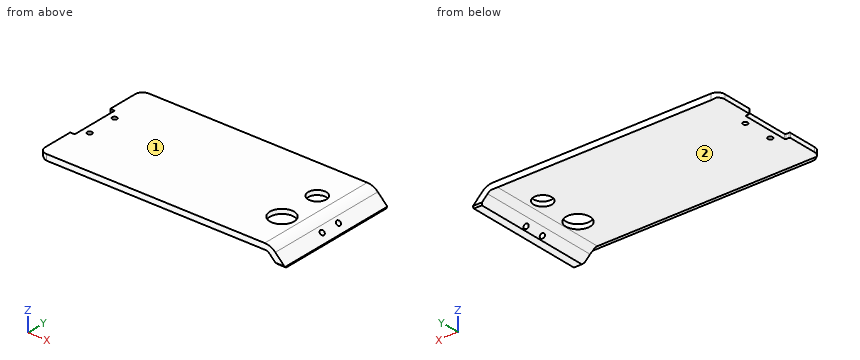
from build123d import *

# Parameters (mm, degrees)
SKETCH_1_W            = 88.2
SKETCH_1_H            = 177
EXTRUDE_1_DEPTH       = 52.9
SHELL_1_T             = -3
CUT_EXTRUDE_5_REACH   = 206.711
SKETCH_16_R           = 6.05
SKETCH_16_R_2         = 8.05
CHAMFER_7_SIZE        = 10
CHAMFER_8_SIZE        = 1
SKETCH_21_W           = 10.5
SKETCH_21_H           = 82.2
EXTRUDE_7_DEPTH       = 6
SKETCH_22_OUTSIDE_W   = 219.942
SKETCH_22_OUTSIDE_H   = 131.142
SKETCH_22_OUTSIDE_W_2 = 164.4
SKETCH_22_OUTSIDE_H_2 = 82
CUT_EXTRUDE_8_DEPTH   = 10
SKETCH_23_W           = 177
SKETCH_23_H           = 42.9
CUT_EXTRUDE_9_DEPTH   = 205.711137948
FILLET_3_R            = 10
FILLET_4_R            = 5.1
SKETCH_24_R           = 1.6
CUT_EXTRUDE_10_DEPTH  = 146.652789194
CHAMFER_10_SIZE       = 1
CHAMFER_10_SIZE_2     = 0.707106781
CUT_EXTRUDE_11_REACH  = 198.013
SKETCH_25_R           = 1.6
FILLET_5_R            = 8
CUT_EXTRUDE_12_REACH  = 198.013
SKETCH_26_W           = 3
SKETCH_26_H           = 32
FILLET_6_R            = 0.5


with BuildPart() as part:
    # 草图1 → 凸台-拉伸1 (new body)
    with BuildSketch(Plane(origin=(0, 0, 0), x_dir=(0, 1, 0), z_dir=(0, 0, 1))):
        with Locations((44.1, -88.5)):
            Rectangle(SKETCH_1_W, SKETCH_1_H)
    extrude(amount=EXTRUDE_1_DEPTH)

    # 抽壳1
    shell_1_openings = [part.faces().sort_by_distance(p)[0] for p in [
        (88.5, 44.1, 0),
    ]]
    offset(amount=SHELL_1_T, openings=shell_1_openings, kind=Kind.INTERSECTION)

    # 草图16 → 切除-拉伸5 (cut, up to next)
    with BuildSketch(Plane.XY.offset(52.9), mode=Mode.PRIVATE) as cut_extrude_5_sk1:
        with Locations((152, 58.2)):
            Circle(SKETCH_16_R)
    cut_extrude_5_tool1 = extrude(cut_extrude_5_sk1.sketch, amount=-CUT_EXTRUDE_5_REACH, mode=Mode.PRIVATE) & part.part
    # 草图16 → 切除-拉伸5 (cut, up to next)
    with BuildSketch(Plane.XY.offset(52.9), mode=Mode.PRIVATE) as cut_extrude_5_sk2:
        with Locations((152, 30)):
            Circle(SKETCH_16_R_2)
    cut_extrude_5_tool2 = extrude(cut_extrude_5_sk2.sketch, amount=-CUT_EXTRUDE_5_REACH, mode=Mode.PRIVATE) & part.part
    add(cut_extrude_5_tool1.solids().sort_by_distance((152, 58.2, 52.9))[0], mode=Mode.SUBTRACT)
    add(cut_extrude_5_tool2.solids().sort_by_distance((152, 30, 52.9))[0], mode=Mode.SUBTRACT)

    # 倒角7
    chamfer_7_edges = [part.edges().sort_by_distance(p)[0] for p in [
        (174, 44.1, 49.9),
        (177, 44.1, 52.9),
    ]]
    chamfer(chamfer_7_edges, length=CHAMFER_7_SIZE)

    # 倒角8
    chamfer_8_edges = [part.edges().sort_by_distance(p)[0] for p in [
        (83.5, 3, 49.9),
        (83.5, 88.2, 52.9),
        (177, 88.2, 21.45),
        (172, 88.2, 47.9),
        (177, 0, 21.45),
        (172, 0, 47.9),
        (83.5, 85.2, 49.9),
        (83.5, 0, 52.9),
    ]]
    chamfer(chamfer_8_edges, length=CHAMFER_8_SIZE)

    # 草图21 → 凸台-拉伸7 (add)
    with BuildSketch(Plane(origin=(0, 0, 0), x_dir=(-1, 0, 0), z_dir=(0, 0, -1))):
        with Locations((-168.75, 44.1)):
            Rectangle(SKETCH_21_W, SKETCH_21_H)
        with Locations((-8.25, 44.1)):
            Rectangle(SKETCH_21_W, SKETCH_21_H)
    extrude(amount=-EXTRUDE_7_DEPTH)

    # 草图22 outside → 切除-拉伸8 (cut)
    with BuildSketch(Plane.XY.offset(52.9)):
        with Locations((88.5, 44.1)):
            Rectangle(SKETCH_22_OUTSIDE_W, SKETCH_22_OUTSIDE_H)
        with Locations((94.8, 44.1)):
            Rectangle(SKETCH_22_OUTSIDE_W_2, SKETCH_22_OUTSIDE_H_2, mode=Mode.SUBTRACT)
    extrude(amount=-CUT_EXTRUDE_8_DEPTH, mode=Mode.SUBTRACT)

    # 草图23 → 切除-拉伸9 (cut, through all)
    with BuildSketch(Plane.XZ):
        with Locations((88.5, 21.45)):
            Rectangle(SKETCH_23_W, SKETCH_23_H)
    extrude(amount=-CUT_EXTRUDE_9_DEPTH, mode=Mode.SUBTRACT)

    # 圆角3
    fillet_3_edges = [part.edges().sort_by_distance(p)[0] for p in [
        (167, 44.1, 52.9),
    ]]
    fillet(fillet_3_edges, radius=FILLET_3_R)

    # 圆角4
    fillet_4_edges = [part.edges().sort_by_distance(p)[0] for p in [
        (12.6, 3.1, 50.95),
        (12.6, 85.1, 50.95),
    ]]
    fillet(fillet_4_edges, radius=FILLET_4_R)

    # 草图24 → 切除-拉伸10 (cut, through all)
    with BuildSketch(Plane(origin=(109.95, 0, 109.95), x_dir=(0.7071067811865456, 0, -0.7071067811865495), z_dir=(0.7071067811865495, 0, 0.7071067811865456))):
        with Locations((88.323019357, 50.6)):
            Circle(SKETCH_24_R)
        with Locations((88.323019357, 37.6)):
            Circle(SKETCH_24_R)
    extrude(amount=-CUT_EXTRUDE_10_DEPTH, mode=Mode.SUBTRACT)

    # 倒角10
    # the kernel refuses this chamfer: 1, 0.707106781 mm, written as the material it takes off along each edge
    with BuildSketch(Plane(origin=(177, 87.671682988, 42.9), x_dir=(-0.6873969152646486, 0, 0.7262819568766976), z_dir=(0, -1, 0))) as chamfer_10_piece_1:
        Polygon((CHAMFER_10_SIZE * 0.999621916911, CHAMFER_10_SIZE * 0.0274958766106), (CHAMFER_10_SIZE_2 * 0.687396915446, CHAMFER_10_SIZE_2 * 0.726281957068), (0, 0), align=None)
    extrude(amount=87.143365976, mode=Mode.SUBTRACT)
    with BuildSketch(Plane(origin=(179.571682988, 3.1, 42.9), x_dir=(0, -0.027495876610586414, 0.9996219169112968), z_dir=(-1, 0, 0))) as chamfer_10_piece_2:
        Polygon((CHAMFER_10_SIZE * 0.999621916911, CHAMFER_10_SIZE * 0.0274958766106), (-CHAMFER_10_SIZE * 0.0274958766106, CHAMFER_10_SIZE * 0.999621916911), (0, 0), align=None)
    extrude(amount=11.143365976, mode=Mode.SUBTRACT)
    with BuildSketch(Plane(origin=(168.428317012, 85.1, 42.9), x_dir=(0, -0.9996219169112968, -0.027495876610589196), z_dir=(1, 0, 0))) as chamfer_10_piece_3:
        Polygon((CHAMFER_10_SIZE * 0.999621916911, -CHAMFER_10_SIZE * 0.0274958766106), (-CHAMFER_10_SIZE * 0.0274958766106, -CHAMFER_10_SIZE * 0.999621916911), (0, 0), align=None)
    extrude(amount=11.143365976, mode=Mode.SUBTRACT)

    # 草图25 → 切除-拉伸11 (cut, up to next)
    with BuildSketch(Plane.XY.offset(52.9), mode=Mode.PRIVATE) as cut_extrude_11_sk1:
        with Locations((20.6, 54.1)):
            Circle(SKETCH_25_R)
    cut_extrude_11_tool1 = extrude(cut_extrude_11_sk1.sketch, amount=-CUT_EXTRUDE_11_REACH, mode=Mode.PRIVATE) & part.part
    # 草图25 → 切除-拉伸11 (cut, up to next)
    with BuildSketch(Plane.XY.offset(52.9), mode=Mode.PRIVATE) as cut_extrude_11_sk2:
        with Locations((20.6, 34.1)):
            Circle(SKETCH_25_R)
    cut_extrude_11_tool2 = extrude(cut_extrude_11_sk2.sketch, amount=-CUT_EXTRUDE_11_REACH, mode=Mode.PRIVATE) & part.part
    add(cut_extrude_11_tool1.solids().sort_by_distance((20.6, 54.1, 52.9))[0], mode=Mode.SUBTRACT)
    add(cut_extrude_11_tool2.solids().sort_by_distance((20.6, 34.1, 52.9))[0], mode=Mode.SUBTRACT)

    # 圆角5
    fillet_5_edges = [part.edges().sort_by_distance(p)[0] for p in [
        (164, 44.1, 49.9),
    ]]
    fillet(fillet_5_edges, radius=FILLET_5_R)

    # 草图26 → 切除-拉伸12 (cut, up to next)
    with BuildSketch(Plane.XY.offset(52.9), mode=Mode.PRIVATE) as cut_extrude_12_sk1:
        with Locations((14.1, 44.1)):
            Rectangle(SKETCH_26_W, SKETCH_26_H)
    cut_extrude_12_tool1 = extrude(cut_extrude_12_sk1.sketch, amount=-CUT_EXTRUDE_12_REACH, mode=Mode.PRIVATE) & part.part
    add(cut_extrude_12_tool1.solids().sort_by_distance((14.1, 44.1, 52.9))[0], mode=Mode.SUBTRACT)

    # 圆角6
    fillet_6_edges = [part.edges().sort_by_distance(p)[0] for p in [
        (12.6, 28.1, 51.4),
        (12.6, 60.1, 51.4),
        (15.6, 60.1, 51.4),
        (15.6, 28.1, 51.4),
    ]]
    fillet(fillet_6_edges, radius=FILLET_6_R)


solid = part.part
Read the model definition and answer for the solid it produces. Units are mm, in the model's axes. Face numbers are marked on the shaded views. Coordinates: 2 decimals unless noted, no trailing zeros. Order: outer loops, then holes, each group sorted by start corner. A loop starts at its lowest first (then second) coordinate and runs counter-clockwise, first axis right, second up. Notation, with made-up numbers: M 86,-19 L 94,-19 A22 ccw 94,-7 Z; hole C 47,-3.75 d4. An arc over 180 degrees is marked long. Put each result on its own line as item: value. Start each with the question number.
Item 1: Consider probe 1 along Y at (x, z) = (20.6, 50.7); probe 2 along Y at (x, z) = (152, 50.55); probe 3 along Z at (x, y) = (81, 20). Determine where each line is inside the solid, lowest interval first. Write a range as [from, to].
Item 2: Given pin 1 Ø2.5 at (x, y) = (20.6, 34.1) entering from +Z; pin 2 Ø1 at (x, z) = (14.5, 51) entering from -Y; pin 3 Ø2.5 at (y, z) = (46.5, 52) entering from -X; pin 4 Ø1.6 at (x, z) = (14, 51) entering from +Y, each flat-ended and moving along its own axis, determine where each tip first touches the part or whether it passes through.
Item 3: Section C-C, the plane y = 54.1 is taken. Determine the outline of the cut face in (x, z).
Item 4: Section D-D, the plane x = 126 is taken. Determine the outline of the cut face in (y, z), plus the area to 3 significant figures.
Item 5: Section B-B, the plane y = 42 is taken. Determine the outline of the cut face in (x, z), plus the area to 3 significant figures.
Item 6: The mould has two halves that part along Y. Classify the marked faces 1 and 2: +Y half, -Y half, draft (parallel to the pull), parting line (faces both ways), or undercut.
Item 7: Section A-A, the plane x = 152 is taken. Determine the outline of the cut face in (y, z).
Computed:
1. probe 1: y = [3.1, 32.5], [35.7, 52.5], [55.7, 85.1]
1. probe 2: y = [3.1, 21.95], [38.05, 52.15], [64.25, 85.1]
1. probe 3: z = [49.9, 52.9]
2. pin 1: passes through
2. pin 2: stops at y = 3.87
2. pin 3: stops at x = 15.6
2. pin 4: stops at y = 84.2
3. outline: M 15.6,49.9 L 19,49.9 L 19,52.9 L 15.6,52.9 Z; M 22.2,49.9 L 147.55,49.9 L 147.55,52.9 L 22.2,52.9 Z; M 156.45,49.9 L 160.69,49.9 A8 cw 166.34,47.56 L 171,42.9 L 176.29,42.9 L 176.29,43.61 L 169.93,49.97 A10 ccw 162.86,52.9 L 156.45,52.9 Z
4. outline: M 3.1,49 L 4,49.9 L 84.2,49.9 L 85.1,49 L 85.1,52.9 L 3.1,52.9 Z
4. area: 247 mm2
5. outline: M 15.6,49.9 L 160.69,49.9 A8 cw 166.34,47.56 L 171,42.9 L 176.29,42.9 L 176.29,43.61 L 169.93,49.97 A10 ccw 162.86,52.9 L 15.6,52.9 Z
5. area: 500 mm2
6. face 1: draft
6. face 2: undercut
7. outline: M 3.1,49 L 4,49.9 L 21.95,49.9 L 21.95,52.9 L 3.1,52.9 Z; M 38.05,49.9 L 52.15,49.9 L 52.15,52.9 L 38.05,52.9 Z; M 64.25,49.9 L 84.2,49.9 L 85.1,49 L 85.1,52.9 L 64.25,52.9 Z
